from build123d import *

# Parameters (mm, degrees)
F0_W     = 210
F0_H     = 50
F1_DEPTH = 12
F2_R     = 3.5
F3_DEPTH = 25
F4_R     = 3.5
F5_DEPTH = 25


# Not quite as in the source:
# - a feature names something its author has since deleted; it is built from what else it names


with BuildPart() as f1:
    # F0 (on Top) → F1 (new body)
    with BuildSketch(Plane.XY):
        with Locations((80.6913864613, -4.2518138885)):
            Rectangle(F0_W, F0_H)
    extrude(amount=F1_DEPTH)

    # F2 (on face) → F3 (cut)
    with BuildSketch(Plane.XY.offset(12)):
        with Locations((119.3913864613, 13.4481861115)):
            Circle(F2_R)
        with Locations((119.3913864613, -21.9518138885)):
            Circle(F2_R)
        with Locations((30.9913864613, -21.9518138885)):
            Circle(F2_R)
        with Locations((-14.0086135387, 13.4481861115)):
            Circle(F2_R)
        with Locations((-14.0086135387, -21.9518138885)):
            Circle(F2_R)
    extrude(amount=-F3_DEPTH, mode=Mode.SUBTRACT)

    # F4 (on face) → F5 (cut)
    with BuildSketch(Plane.XY.offset(12)):
        with Locations((30.6913864613, 13.4481861115)):
            Circle(F4_R)
    extrude(amount=-F5_DEPTH, mode=Mode.SUBTRACT)


solid = f1.part
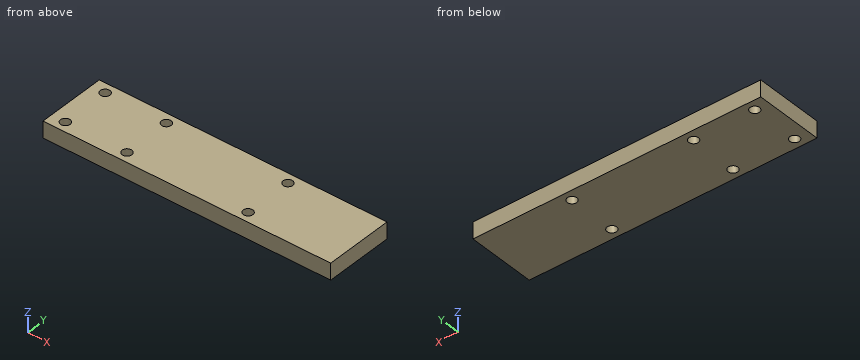
Design review of the part built by this model. Coordinates are the model's own, in mm. Give positions to 0.01 mm unless a question says otherwise; leave off trailing zeros. Order: outer loops, then holes, each group sorted by start corner. A loop starts at its lowest first (then second) coordinate and runs counter-clockwise, first axis right, second up.
1. Add section A-A, the plane z = 9.75. State the section outline as (x, y) points.
Solution:
outline: (-24.31, -29.25) - (185.69, -29.25) - (185.69, 20.75) - (-24.31, 20.75) - close; hole circle Ø7 at (-14.01, -21.95); hole circle Ø7 at (-14.01, 13.45); hole circle Ø7 at (30.69, 13.45); hole circle Ø7 at (30.99, -21.95); hole circle Ø7 at (119.39, -21.95); hole circle Ø7 at (119.39, 13.45)
2. For pin 1 Ø3 at (x, y) = (49.5, -18.5) entering from -Z, flat-tipped, find the tip position at first contact; note if it passes through.
Solution:
pin 1: stops at z = 0
3. To check wall thickness, follow L1, parallel to X at y = 13.5, z = 10; L2, parallel to X at y = -21, z = 9.5; L3, parallel to Y at x = 28.5, z = 3. State the ranges of each line that lie inside material, in increasing order.
Solution:
L1: x = -24.31 to -17.51, -10.51 to 27.19, 34.19 to 115.89, 122.89 to 185.69
L2: x = -24.31 to -17.38, -10.64 to 27.62, 34.36 to 116.02, 122.76 to 185.69
L3: y = -29.25 to -24.41, -19.49 to 10.72, 16.18 to 20.75
